Autodesk Inventor part; units mm, degrees
ref_plane "YZ Plane" through (0, 0, 0) normal (1, 0, 0) x (0, 1, 0)
ref_plane "XZ Plane" through (0, 0, 0) normal (0, 1, 0) x (-1, 0, 0)
ref_plane "XY Plane" through (0, 0, 0) normal (0, 0, 1) x (1, 0, 0)
sketch "Sketch1" plane through (0, 0, 0) normal (0, 0, 1) x (1, 0, 0)
  line L0 (0, 0) -> (190.5, 0)
  line L1 (190.5, 0) -> (190.5, 635)
  line L2 (190.5, 635) -> (0, 635)
  line L3 (0, 635) -> (0, 0)
  dimension "d0" = 190.5
  dimension "d1" = 635
extrude "Extrusion1" add sketch "Sketch1" along normal blind 3.175
sketch "Sketch2" plane through (0, 0, 3.175) normal (0, 0, 1) x (1, 0, 0)
  line L0 (0, 0) -> (0, 635)
  line L1 (190.5, 0) -> (0, 0)
  line L2 (165.1, 0) -> (0, 0)
  line L3 (0, 88.9) -> (165.1, 0)
  line L4 (0, 635) -> (190.5, 635)
  line L5 (165.1, 635) -> (0, 635)
  line L6 (0, 457.2) -> (165.1, 635)
  line L7 (0, 457.2) -> (0, 635)
  line L8 (165.1, 635) -> (165.1, 0) construction
  line L9 (190.5, 635) -> (190.5, 0)
  dimension "d5" = 88.9
  dimension "d8" = 177.8
  dimension "d9" = 25.4
extrude "Extrusion2" cut sketch "Sketch2" against normal up to next contours L0 L3 L1 | L0 L4 L6
sketch "Sketch4" plane through (0, 0, 3.175) normal (0, 0, 1) x (1, 0, 0)
  line L0 (0, 88.9) -> (0, 457.2)
  line L1 (0, 330.2) -> (50.8, 330.2)
  line L2 (50.8, 330.2) -> (50.8, 127)
  line L3 (50.8, 127) -> (0, 127)
  line L4 (0, 127) -> (0, 330.2)
  line L5 (165.1, 635) -> (50.8, 635) construction
  line L6 (50.8, 635) -> (50.8, 330.2) construction
  line L7 (50.8, 127) -> (50.8, 0) construction
  line L8 (50.8, 0) -> (165.1, 0) construction
  point P0 (0, 0)
  dimension "d17" = 203.2
  dimension "d18" = 50.8
  dimension "d21" = 127
extrude "Extrusion4" cut sketch "Sketch4" against normal through all
properties part number "Conveyor_Frame_BottomStabilizerPlate" material "Aluminum-6061"
Verification items for the finished model (mm, model axes). Round coordinates to 2 decimals unless told otherwise and drop trailing zeros. Order: outer loops, then holes, each group sorted by start corner. A loop starts at its lowest first (then second) coordinate and runs counter-clockwise, first axis right, second up. Notation, with made-up numbers: (-5.5, -21.5) -> (53.5, -21.5) arc R14 cw to (53.5, -7.5) -> close; hole circle Ø6 at (85, -17). An arc over 180 degrees is marked (long way). Put each result on its own line as item: value. Start each with the question number.
(1) Section check D-D (x = 90). Enter the section's corners in (y, z) (3 decimals), then the cut area to 3 significant figures.
(2) Material ranges on line 1 along X through (y, z) = (260, 2.35); line 2 along Y through (x, z) = (29, 0.85); line 3 along Y through (x, z) = (165, 2.85), recorded low to high.
(3) Section check A-A (x = 19.5). Enter the section's corners in (y, z) (3 decimals), then the cut area to 3 significant figures.
(4) Section check B-B (z = 2.15). Enter the section's corners in (x, y).
(5) Depth check by flat-ended pin: pin 1 Ø4 at (x, y) = (69.5, 326) entering from -Z; pin 2 Ø1.6 at (x, z) = (35.5, 2) entering from -Y. Enter the tip coordinate at first touch or a pass-through.
(6) Section check C-C (y = 307). Enter the section's corners in (x, z) (3 decimals), then the cut area to 3 significant figures.
Completed:
1. outline: (40.438, 0) -> (554.123, 0) -> (554.123, 3.175) -> (40.438, 3.175) -> close
1. area: 1,630 mm2
2. line 1: x = 50.8 to 190.5
2. line 2: y = 73.28 to 127, 330.2 to 488.43
2. line 3: y = 0.05 to 634.89
3. outline: (78.4, 0) -> (127, 0) -> (127, 3.175) -> (78.4, 3.175) -> close; (330.2, 0) -> (478.2, 0) -> (478.2, 3.175) -> (330.2, 3.175) -> close
3. area: 624 mm2
4. outline: (0, 88.9) -> (165.1, 0) -> (190.5, 0) -> (190.5, 635) -> (165.1, 635) -> (0, 457.2) -> (0, 330.2) -> (50.8, 330.2) -> (50.8, 127) -> (0, 127) -> close
5. pin 1: stops at z = 0
5. pin 2: stops at y = 69.35
6. outline: (50.8, 0) -> (190.5, 0) -> (190.5, 3.175) -> (50.8, 3.175) -> close
6. area: 444 mm2
